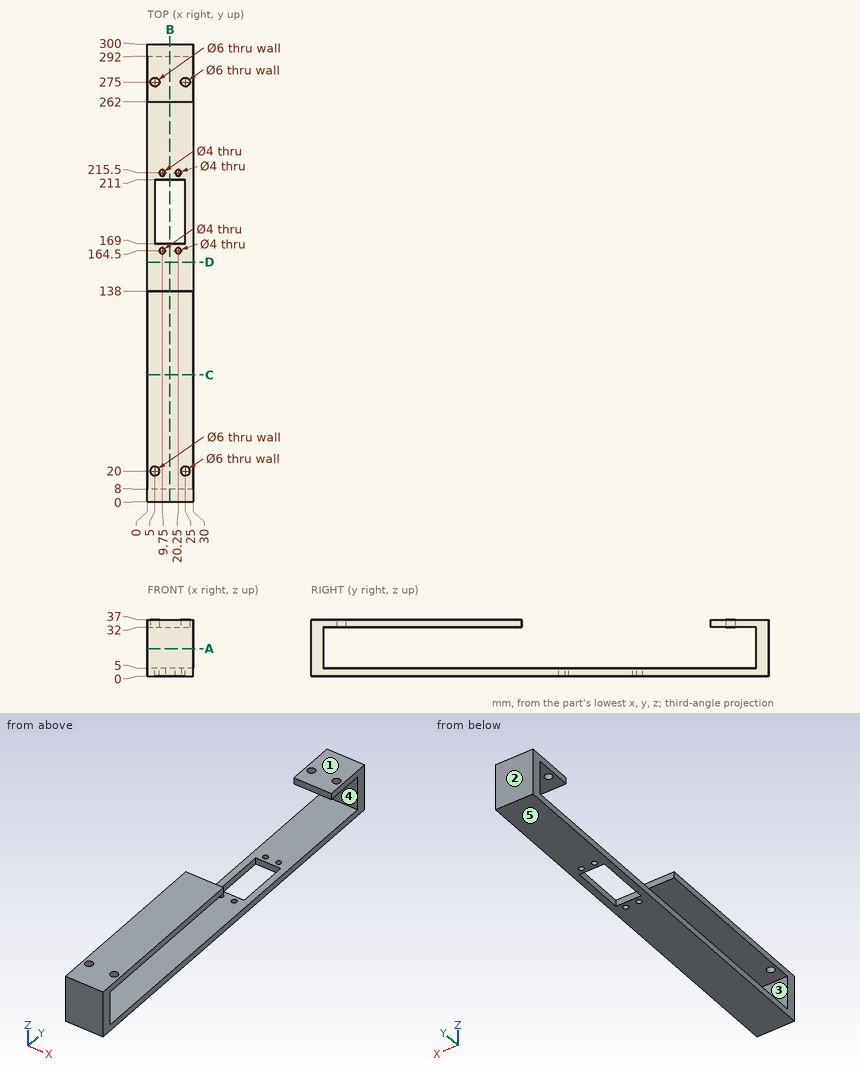
Input: dimensioned drawing with shaded views. Units: mm. Origin: part minimum x, y, z. A direction names the side the tool comes from. Give positions to 0.01 mm unless a question says otherwise; leave off trailing zeros. Loops run counter-clockwise (first coordinate to the right, second up) from the corner with the lowest first, then second, coordinate; pieces in that order, holes last. Notation, with made-up numbers: (86, 41.25) -> (119, 41.25) arc R18 cw to (119, 60.25) -> close; hole circle Ø4 at (-5.75, -5.5). An arc over 180 degrees is marked (long way). Use a Markdown table: item, result. Add a question column.
1) Reachability of the marked faces 4 and 5 from +Z, -Z, +X, -X, +Y, -Y: full face, straight path, thin tool, end or side. Return the list, or none.
2) Section query C-C, the plane y = 83. Return the cut outline in (x, z), then the cut area to 3 significant figures.
3) Section query B-B, the plane x = 14.75. Return the cut outline in (y, z).
4) Pull-direction query (Y, two-part tool) for the marked faces 1, 2 and 3; classes: +Y half, -Y half, draft (parallel to the pull), parting line (faces both ways), or undercut.
5) Section query A-A, the plane z = 18. Return the cut outline in (x, y), then the cut area to 3 significant figures.
6) Section query D-D, the plane y = 157. Return the cut outline in (x, z), then the cut area to 3 significant figures.
7) First-contact query: pin 1 (10 mm diameter, centred on x = 17, z = 26, fed in from -Y); pin 2 (3 mm diameter, centred on x = 20.25, y = 164.5, fed in from +Z); pin 3 (5 mm diameter, centred on x = 9.75, y = 215.5, fed in from +Z). Flat tips, straight axial feed; report the tip coordinate or a pass-through.
8) Line query: line 1 along X through (y, z) = (215.5, 2.3); line 2 along Y through (x, z) = (4.75, 35); line 3 along Y through (x, z) = (9.75, 3.2). Output: solid intervals per line, ascending. Write a range as [from, to].
Numbers:
| question | item | result |
|---|---|---|
| 1 | face 4 | +X, -X |
| 1 | face 5 | -Z, +X, -X, +Y, -Y |
| 2 | outline | (0, 0) -> (30, 0) -> (30, 5) -> (0, 5) -> close; (0, 32) -> (30, 32) -> (30, 37) -> (0, 37) -> close |
| 2 | area | 300 mm2 |
| 3 | outline | (0, 0) -> (169, 0) -> (169, 5) -> (8, 5) -> (8, 32) -> (138, 32) -> (138, 37) -> (0, 37) -> close; (211, 0) -> (300, 0) -> (300, 37) -> (262, 37) -> (262, 32) -> (292, 32) -> (292, 5) -> (211, 5) -> close |
| 4 | face 1 | draft |
| 4 | face 2 | +Y half |
| 4 | face 3 | undercut |
| 5 | outline | (0, 0) -> (30, 0) -> (30, 8) -> (0, 8) -> close; (0, 292) -> (30, 292) -> (30, 300) -> (0, 300) -> close |
| 5 | area | 480 mm2 |
| 6 | outline | (0, 0) -> (30, 0) -> (30, 5) -> (0, 5) -> close |
| 6 | area | 150 mm2 |
| 7 | pin 1 | stops at y = 0 |
| 7 | pin 2 | passes through |
| 7 | pin 3 | stops at z = 5 |
| 8 | line 1 | x = [0, 7.75], [11.75, 18.25], [22.25, 30] |
| 8 | line 2 | y = [0, 17.01], [22.99, 138], [262, 272.01], [277.99, 300] |
| 8 | line 3 | y = [0, 162.5], [166.5, 169], [211, 213.5], [217.5, 300] |
